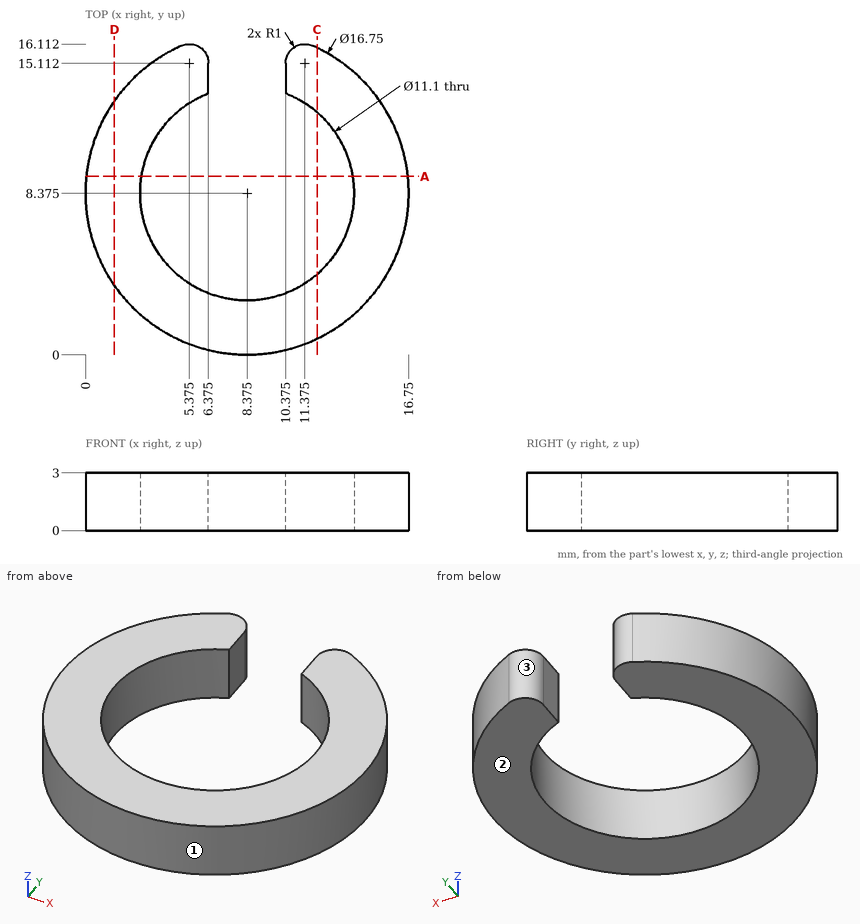
Check sheet for the drawn part. Datum: minimum x, y, z corner. Units: mm. Give positions to 0.01 mm unless a question says otherwise; leave off trailing zeros. Write each loop counter-clockwise with the first axis right and the second up, starting at its lowest first coordinate (ties: lowest second). Pieces come first, ordered by that corner, then holes. Notation, with made-up numbers: M 43,14.25 L 53,14.25 A22 cw 53,40.25 Z; hole C -39.75,73 d3. An arc over 180 degrees is marked long. One line per question, with ' | ' between items.
1) Gauge pin test, flat ends, axial feed: pin 1 Ø6 at (x, y) = (6, 5) entering from -Z; pin 2 Ø0.5 at (y, z) = (14.5, 1.5) entering from -X; pin 3 Ø1.2 at (y, z) = (14, 2) entering from +X (1 decimal). Record the tip position at first contact, or that the pin passes through.
Result:
pin 1: stops at z = 0 | pin 2: stops at x = 2.41 | pin 3: stops at x = 15.1
2) Thickness scan on line 1 along X through (y, z) = (11.5, 1.4) (1 decimal); line 2 along Y through (x, z) = (5.75, 1.35) (1 decimal); line 3 along X through (y, z) = (11, 1.25) (1 decimal). Record the ranges inside material, lowest first. Write a range as [from, to].
Result:
line 1: x = [0.6, 3.8], [13, 16.1] | line 2: y = [0.4, 3.5], [13.3, 16] | line 3: x = [0.4, 3.5], [13.3, 16.3]
3) Section check C-C on x = 12. Enter the section's corners in (y, z) (1 decimal), plus the area to 3 significant figures.
Result:
outline: M 0.8,0 L 4.2,0 L 4.2,3 L 0.8,3 Z; M 12.6,0 L 15.9,0 L 15.9,3 L 12.6,3 Z | area: 20.1 mm2
4) Section check D-D on x = 1.5. Enter the section's corners in (y, z).
Result:
outline: M 3.59,0 L 13.16,0 L 13.16,3 L 3.59,3 Z
5) Mould release check, pull along X, two halves, no side actions. Record for the marked faces 1, 2 and 3: released by +X, released by -X, zero draft, split by the parting line, or undercut.
Result:
face 1: split by the parting line | face 2: zero draft | face 3: undercut
6) Section check A-A on y = 9.25. Enter the section's corners in (x, z), plus the area to 3 significant figures.
Result:
outline: M 0.05,0 L 2.89,0 L 2.89,3 L 0.05,3 Z; M 13.86,0 L 16.7,0 L 16.7,3 L 13.86,3 Z | area: 17.1 mm2
